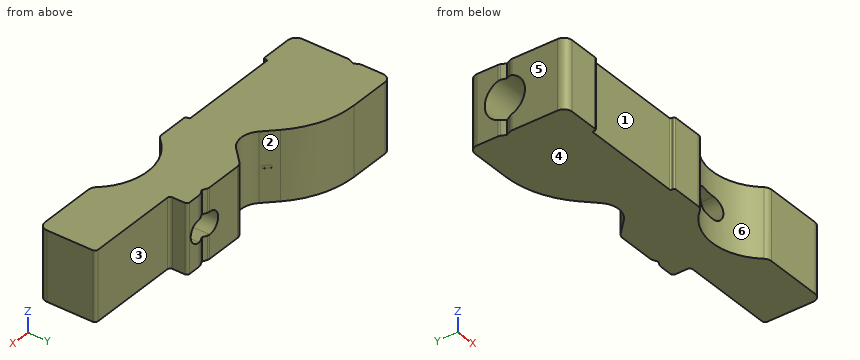
```python
from build123d import *

# Parameters (mm, degrees)
PAD_DEPTH            = 12.5
SKETCH001_R          = 10.1
POCKET_DEPTH         = 0.5
SKETCH002_R          = 7.25
HOLE_DEPTH           = 30.643761
HOLE_TIPS_R          = 7.25
POCKET001_DEPTH      = 35.001
POCKET001_DEPTH_BACK = 0.001


with BuildPart() as part:
    # Sketch → Pad (new body, symmetric)
    with BuildSketch(Plane.XY):
        with BuildLine():
            Line((0, 32), (0, 24.5))
            ThreePointArc((0, 24.5), (0.047408, 24.067121), (0.187384, 23.654763))
            Line((0.187384, 23.654763), (0.959013, 22))
            Line((0.959013, 22), (0.187384, 20.345237))
            ThreePointArc((0.187384, 20.345237), (0.047408, 19.932879), (0, 19.5))
            Line((0, 3), (0, 19.5))
            ThreePointArc((0, 3), (0.87868, 0.87868), (3, 0))
            Line((3, 0), (14, 0))
            ThreePointArc((14, 0), (14.353553, 0.146447), (14.5, 0.5))
            Line((14.5, 1), (14.5, 0.5))
            ThreePointArc((15, 1.5), (14.646447, 1.353553), (14.5, 1))
            Line((15, 1.5), (51, 1.5))
            ThreePointArc((51.5, 1), (51.353553, 1.353553), (51, 1.5))
            Line((51.5, 1), (51.5, 0.5))
            ThreePointArc((51.5, 0.5), (51.646447, 0.146447), (52, 0))
            Line((52, 0), (62.564404, 0))
            ThreePointArc((62.564404, 0), (63.815491, 0.27332), (64.838612, 1.043478))
            ThreePointArc((95.161388, 1.043478), (80, 8), (64.838612, 1.043478))
            ThreePointArc((95.161388, 1.043478), (96.184509, 0.27332), (97.435596, 0))
            Line((97.435596, 0), (118, 0))
            ThreePointArc((118, 0), (120.12132, 0.87868), (121, 3))
            Line((121, 19.5), (121, 3))
            ThreePointArc((121, 19.5), (120.707107, 20.207107), (120, 20.5))
            Line((87, 20.5), (120, 20.5))
            ThreePointArc((86, 21.5), (86.292893, 20.792893), (87, 20.5))
            Line((86, 26), (86, 21.5))
            ThreePointArc((86, 26), (85.707107, 26.707107), (85, 27))
            Line((80.5, 27), (85, 27))
            ThreePointArc((80.5, 27), (80.067121, 26.952592), (79.654763, 26.812616))
            Line((78, 26.040987), (79.654763, 26.812616))
            Line((76.345237, 26.812616), (78, 26.040987))
            ThreePointArc((76.345237, 26.812616), (75.932879, 26.952592), (75.5, 27))
            Line((62.384776, 27), (75.5, 27))
            ThreePointArc((62.384776, 27), (61.236726, 26.771639), (60.263456, 26.12132))
            Line((60.263456, 26.12132), (55.363961, 21.221825))
            ThreePointArc((44.636039, 21.221825), (50, 19), (55.363961, 21.221825))
            Line((40.230447, 25.627417), (44.636039, 21.221825))
            ThreePointArc((40.230447, 25.627417), (29.8489, 32.564145), (17.60303, 35))
            Line((3, 35), (17.60303, 35))
            ThreePointArc((3, 35), (0.87868, 34.12132), (0, 32))
        make_face()
    extrude(amount=PAD_DEPTH, both=True)

    # Sketch001 → Pocket (cut, symmetric)
    with BuildSketch(Plane.XY):
        with Locations((50, 30)):
            Circle(SKETCH001_R)
    extrude(amount=POCKET_DEPTH, both=True, mode=Mode.SUBTRACT)

    # Sketch002 → Hole (cut)
    with BuildSketch(Plane.YZ):
        with Locations((22, 0)):
            Circle(SKETCH002_R)
    extrude(amount=HOLE_DEPTH, mode=Mode.SUBTRACT)

    # Hole tips → Hole tip 1 section 0
    with BuildSketch(Plane.YZ.offset(30.643761), mode=Mode.PRIVATE) as hole_tip_1_s0:
        with Locations((22, 0)):
            Circle(HOLE_TIPS_R)
    loft([hole_tip_1_s0.sketch, Vertex(35, 22, 0)], mode=Mode.SUBTRACT)

    # Sketch003 → Pocket001 (cut, two sides)
    with BuildSketch(Plane.XZ) as pocket001_sk:
        with BuildLine():
            ThreePointArc((75.5, 4), (71.5, 0), (75.5, -4))
            Line((75.5, -4), (80.5, -4))
            ThreePointArc((80.5, -4), (84.5, 0), (80.5, 4))
            Line((75.5, 4), (80.5, 4))
        make_face()
    extrude(amount=-POCKET001_DEPTH, mode=Mode.SUBTRACT)
    extrude(pocket001_sk.sketch, amount=POCKET001_DEPTH_BACK, mode=Mode.SUBTRACT)


solid = part.part
```
The model under review builds one solid part; all positions refer to its coordinate system, in mm. Face numbers are marked on the shaded views. A direction names the side the tool comes from. Coordinates: 2 decimals unless noted, no trailing zeros. Order: outer loops, then holes, each group sorted by start corner. A loop starts at its lowest first (then second) coordinate and runs counter-clockwise, first axis right, second up. Notation, with made-up numbers: (46, 19.25) -> (88, 19.25) arc R24 cw to (88, 54.25) -> close; hole circle Ø1 at (34, 79). An arc over 180 degrees is marked (long way). Answer in a Markdown table with one row per item. Add a question column.
Item 1: We need section A-A on y = 12.5. Write out the cut boundary in (x, z).
Item 2: Mouldability with a two-part tool opening along X and no side actions: class the marked faces 4, 5 and 6 as +X half, -X half, draft (parallel to the pull), parting line (faces both ways), or undercut.
Item 3: To check wall thickness, follow probe 1 along Z at (x, y) = (16.5, 22); probe 2 along Y at (x, z) = (108, -1.5); probe 3 along X at (y, z) = (11, 1). State the ranges of each line that lie inside material, in increasing order.
Item 4: We need section C-C on y = 5. Write out the cut boundary in (x, z).
Item 5: Machinability: for the marked faces 1, 2 and 3, which of the approach directions +Z, -Z, +X, -X, +Y, -Y give a long, thin tool a straight path to every point of the face, cutting with its end or side? Answer none if there is none.
Item 6: We need section D-D on x = 99. Write out the cut boundary in (y, z), plus the area to 4 significant figures.
Item 7: Clearance check with flat-ended pins moving along their axes: pin 1 (10.5 mm diameter, centred on x = 69.5, z = -4.5, fed in from +Y); pin 2 (7.5 mm diameter, centred on x = 97.5, z = -3, fed in from +Y); pin 3 (3 mm diameter, centred on x = 29.5, z = 9.5, fed in from +Y). State where each tip first meets the part, or that it passes through.
Item 8: We need section B-B on x = 9. Write out the cut boundary in (y, z), plus the area to 3 significant figures.
Final values:
| question | item | result |
|---|---|---|
| 1 | outline | (0, -12.5) -> (121, -12.5) -> (121, 12.5) -> (0, 12.5) -> close; hole (75.5, -4) -> (80.5, -4) arc R4 ccw to (80.5, 4) -> (75.5, 4) arc R4 ccw to start |
| 2 | face 4 | draft |
| 2 | face 5 | -X half |
| 2 | face 6 | undercut |
| 3 | probe 1 | z = -12.5 to -7.25, 7.25 to 12.5 |
| 3 | probe 2 | y = 0 to 20.5 |
| 3 | probe 3 | x = 0 to 71.63, 84.37 to 121 |
| 4 | outline | (0, -12.5) -> (69.46, -12.5) -> (69.46, 12.5) -> (0, 12.5) -> close; (90.54, -12.5) -> (121, -12.5) -> (121, 12.5) -> (90.54, 12.5) -> close |
| 5 | face 1 | +Z, -Z, -Y |
| 5 | face 2 | +Z, -Z, +Y |
| 5 | face 3 | +Z, -Z, +X, +Y |
| 6 | outline | (0, -12.5) -> (20.5, -12.5) -> (20.5, 12.5) -> (0, 12.5) -> close |
| 6 | area | 512.5 mm2 |
| 7 | pin 1 | stops at y = 27 |
| 7 | pin 2 | stops at y = 20.5 |
| 7 | pin 3 | stops at y = 33.26 |
| 8 | outline | (0, -12.5) -> (35, -12.5) -> (35, 12.5) -> (0, 12.5) -> close; hole circle Ø14.5 at (22, 0) |
| 8 | area | 710 mm2 |
